The model under review builds one solid part; all positions refer to its coordinate system, in mm. A direction names the side the tool comes from. Round coordinates to 2 decimals unless told otherwise and drop trailing zeros. Order: outer loops, then holes, each group sorted by start corner. A loop starts at its lowest first (then second) coordinate and runs counter-clockwise, first axis right, second up. Notation, with made-up numbers: M 85,59 L 102,59 A22 ccw 102,76 Z; hole C 80.5,-39.75 d11. An arc over 180 degrees is marked long. Use a Markdown table: item, result. Add a question column.
1. Consider section A-A on z = 16.5. State the section outline as (x, y) points.
2. To check wall thickness, follow probe 1 along X at (y, z) = (0.65, -4.5); probe 2 along Z at (x, y) = (-7, 0.55); probe 3 along Z at (x, y) = (-8.5, 0.75). State the ranges of each line that lie inside material, in increasing order.
3. For faces 1 (the cylindrical face through (20, 1, 48)), 2 (the flat face through (16, 0, 5)), list the 3-axis set-ups (+Z, -Z, +X, -X, +Y, -Y) from which the entire face can be reached by the end or side of a thin tool; tool diameter is ignored.
4. Consider section D-D on z = -57.5. State the section outline as (x, y) points, then the cut area to 3 significant figures.
5. Consider section B-B on z = 0. State the section outline as (x, y) points, then the cut area to 3 significant figures.
6. Consider section C-C on y = 1.55. Count the separate pieces of the cut face and the enclosed holes in it, then the cut area to 3 significant figures.
7. The part is to be moulded in two halves that separate along Z. For faces 3 (the cylindrical face through (30.059, 0.986, 44.155)), 4 (the cylindrical face through (31.97, 1.01, 2.87)), 5 (the flat face through (16, 2, 5)), say which applies: +Z half, -Z half, draft (parallel to the pull), parting line (faces both ways), or undercut.
from build123d import *

# Parameters (mm, degrees)
SKETCH_1_R          = 1.65
SKETCH_1_R_2        = 5.5
EXTRUDE_1_DEPTH     = 2
SKETCH_2_R          = 1.65
CUT_EXTRUDE_1_DEPTH = 85.204030668
FILLET_1_R          = 2
FILLET_2_R          = 12


with BuildPart() as part:
    # Эскиз1 → Бобышка-Вытянуть1 (new body)
    with BuildSketch(Plane(origin=(0, 0, 0), x_dir=(1, 0, 0), z_dir=(0, 1, 0))):
        with BuildLine():
            Line((-7.358068948, -9.479389292), (-18.08780174, -24.976764467))
            ThreePointArc((-18.08780174, -24.976764467), (-19.487318719, -47.710015139), (0, -59.5))
            ThreePointArc((0, -59.5), (22.769664226, -54.970832184), (42.072853481, -42.072853481))
            ThreePointArc((42.072853481, -42.072853481), (47.515690449, -19.956460022), (30.451246794, -4.87123226))
            Line((30.451246794, -4.87123226), (28.075866666, 35.356540564))
            ThreePointArc((28.075866666, 35.356540564), (24.846341863, 51.541564262), (17.329317504, 66.234391334))
            ThreePointArc((17.329317504, 66.234391334), (8.97294662, 67.707844982), (7.499492972, 59.351474098))
            ThreePointArc((7.499492972, 59.351474098), (16.145431017, 33.64630977), (9.479389292, 7.358068948))
            ThreePointArc((9.479389292, 7.358068948), (-8.485281374, 8.485281374), (-7.358068948, -9.479389292))
        make_face()
        with Locations(Location((10.729446295, -53.940569088, 0), (0, 0, 270))):
            Circle(SKETCH_1_R, mode=Mode.SUBTRACT)
        with Locations(Location((30.554877949, -45.728606417, 0), (0, 0, 90))):
            Circle(SKETCH_1_R, mode=Mode.SUBTRACT)
        with Locations(Location((0, 0, 0), (0, 0, 270))):
            Circle(SKETCH_1_R_2, mode=Mode.SUBTRACT)
        with Locations(Location((0, -9, 0), (0, 0, 270))):
            Circle(SKETCH_1_R, mode=Mode.SUBTRACT)
        with Locations(Location((-7.794228634, 4.5, 0), (0, 0, 270))):
            Circle(SKETCH_1_R, mode=Mode.SUBTRACT)
        with Locations(Location((7.794228634, 4.5, 0), (0, 0, 270))):
            Circle(SKETCH_1_R, mode=Mode.SUBTRACT)
        with BuildLine():
            Line((-5.548909769, -24.103746779), (20.967594525, -13.120251073))
            ThreePointArc((20.967594525, -13.120251073), (38.572813673, -18.460735916), (36.769552622, -36.769552622))
            ThreePointArc((36.769552622, -36.769552622), (19.899538483, -48.041735691), (0, -52))
            ThreePointArc((0, -52), (-14.221386566, -40.328809669), (-5.548909769, -24.103746779))
        make_face(mode=Mode.SUBTRACT)
    extrude(amount=EXTRUDE_1_DEPTH)

    # Эскиз2 → Вырез-Вытянуть1 (cut, through all)
    with BuildSketch(Plane.XZ):
        with Locations(Location((21.974708544, -27.113395045, 0), (0, 0, 270))):
            Circle(SKETCH_2_R)
        with Locations(Location((12.414405238, -62.792932716, 0), (0, 0, 270))):
            Circle(SKETCH_2_R)
        with Locations(Location((20.340189466, -45.796033589, 0), (0, 0, 270))):
            Circle(SKETCH_2_R)
    extrude(amount=-CUT_EXTRUDE_1_DEPTH, mode=Mode.SUBTRACT)

    # Скругление1
    fillet_1_edges = [part.edges().sort_by_distance(p)[0] for p in [
        (-7.358068948, 1, 9.479389292),
        (9.479389292, 1, -7.358068948),
    ]]
    fillet(fillet_1_edges, radius=FILLET_1_R)

    # Скругление2
    fillet_2_edges = [part.edges().sort_by_distance(p)[0] for p in [
        (30.451246794, 1, 4.87123226),
    ]]
    fillet(fillet_2_edges, radius=FILLET_2_R)


solid = part.part
Answer block:
| question | item | result |
|---|---|---|
| 1 | outline | M -12.22,0 L 12.81,0 L 12.81,2 L -12.22,2 Z; M 37,0 L 46.1,0 L 46.1,2 L 37,2 Z |
| 2 | probe 1 | -11.12 to -9.44, -6.14 to -3.16, 3.16 to 6.14, 9.44 to 29.9 |
| 2 | probe 2 | -9.75 to -5.95, -3.05 to 24.8, 50.2 to 58.36 |
| 2 | probe 3 | -8.47 to -5.99, -3.01 to 8.48, 11.13 to 25.75, 49.25 to 57.79 |
| 3 | face 1 | +Y, -Y |
| 3 | face 2 | +Z, -Z, +X, -X, -Y |
| 4 | outline | M 8.73,0 L 22.41,0 L 22.41,2 L 8.73,2 Z |
| 4 | area | 27.3 mm^2 |
| 5 | outline | M -12,0 L -5.5,0 L -5.5,2 L -12,2 Z; M 5.5,0 L 30.57,0 L 30.57,2 L 5.5,2 Z |
| 5 | area | 63.1 mm^2 |
| 6 | separate pieces | 1 |
| 6 | enclosed holes | 10 |
| 6 | area | 2,740 mm^2 |
| 7 | face 3 | undercut |
| 7 | face 4 | -Z half |
| 7 | face 5 | draft |
